from build123d import *

# Parameters (mm, degrees)
FILLET1_R = 7.62


with BuildPart() as part:
    # Sketch2 → Revolve1 (revolve)
    with BuildSketch(Plane.XY):
        Polygon((-58.2676, 43.2769703), (-58.2676, 40.2035703), (-60.12897926, 36.239383837), (-57.831323448, 26.163828165), (-62.828989293, 36.465258256), (-60.8076, 40.770218692), (-60.8076, 42.829099769), (-64.137873862, 51.978952006), (-60.8076, 60.025592649), (-60.8076, 64.821818572), (-73.025, 72.733281474), (-58.2676, 66.631684467), (-58.2676, 60.025592649), (-61.3156, 51.651281474), align=None)
    revolve(axis=Axis((0, 0, 0), (0, 1, 0)))

    # Fillet1
    fillet1_edges = [part.edges().sort_by_distance(p)[0] for p in [
        (64.137873862, 51.978952006, 0),
        (60.8076, 42.829099769, 0),
        (62.828989293, 36.465258256, 0),
        (60.8076, 64.821818572, 0),
    ]]
    fillet(fillet1_edges, radius=FILLET1_R)


solid = part.part
Build history of the part. All positions in model axes, mm. A direction names the side the tool comes from. Coordinates: 2 decimals unless noted, no trailing zeros.
(1) Pin check, flat tips, straight feed: pin 1 Ø6 at (x, y) = (49.5, 46) entering from +Z; pin 2 Ø3 at (y, z) = (43, -3.5) entering from -X; pin 3 Ø1 at (y, z) = (50.5, -1) entering from +X. Stop position of each tip, or through.
(2) Mould opens along Y. For faces 1 (the conical face through (64.77, 67.43, 2.85)), 2 (the cylindrical face through (12.631, 63.282, -56.882)), 3 (the conical face through (12.657, 39.956, -56.996)) say: pulls with the +Y half, pulls with the -Y half, needs draft (parallel to the pull), parting line crosses it, or undercut.
(3) Drill centre lines: line 1 (Z direction, x = 0, y = 63.5); line 2 (Z direction, x = 0, y = 41.5); line 3 (X direction, y = 54, z = -16). Where is each one in solid material? Low to high.
(4) 3-axis set-ups, long thin cutter, end or side, ignore diameter. For faces 4 (the cylindrical face through (12.631, 41.719, -56.882)), 5 (the cylindrical face through (-58, 41.13, 18.26)): which of +Z, -Z, +X, -X, +Y, -Y reach the whole face in a straight line?
Working result:
1. pin 1: stops at z = 41.33
1. pin 2: stops at x = -61.32
1. pin 3: stops at x = 63.53
2. face 1: pulls with the -Y half
2. face 2: needs draft
2. face 3: undercut
3. line 1: z = -61.35 to -58.27, 58.27 to 61.35
3. line 2: z = -60.81 to -58.27, 58.27 to 60.81
3. line 3: x = -61.2 to -58.31, 58.31 to 61.2
4. face 4: +Y
4. face 5: none
